Check sheet for the modelled part. Datum: model origin and axes. Units: mm. A direction names the side the tool comes from. Give positions to 0.01 mm unless a question says otherwise; leave off trailing zeros. Order: outer loops, then holes, each group sorted by start corner. A loop starts at its lowest first (then second) coordinate and runs counter-clockwise, first axis right, second up. Notation, with made-up numbers: (76, 4) -> (104, 4) arc R21 cw to (104, 13) -> close; hole circle Ø5 at (2, -5). An arc over 180 degrees is marked (long way). One line per question, with ' | ' between items. Start each with the question number.
from build123d import *

# Parameters (mm, degrees)
EXTRUDE_1_DEPTH      = 2
SKETCH_2_R           = 2.75
CUT_EXTRUDE_1_DEPTH  = 76.957158978
EXTRUDE_2_DEPTH      = 32
EXTRUDE_2_DEPTH_BACK = 2
SKETCH_3_W           = 22.737902435
SKETCH_3_H           = 2
CUT_EXTRUDE_2_DEPTH  = 83.398361634
SKETCH_7_W           = 1
SKETCH_7_H           = 2
CUT_EXTRUDE_3_DEPTH  = 2
FILLET_1_R           = 3
FILLET_2_R           = 1


with BuildPart() as part:
    # 草图1 → 凸台-拉伸1 (new body)
    with BuildSketch(Plane(origin=(0, 0, 0), x_dir=(1, 0, 0), z_dir=(0, 1, 0))):
        Polygon((0, 0), (39.728252902, 0), (70.5, -11.2), (70.5, -28.2), (35.853451717, -28.2), (0, -7.5), align=None)
    extrude(amount=EXTRUDE_1_DEPTH)

    # 草图2 → 切除-拉伸1 (cut, through all)
    with BuildSketch(Plane(origin=(0, 2, 0), x_dir=(1, 0, 0), z_dir=(0, 1, 0))):
        with Locations(Location((59, -16.7, 0), (0, 0, 270))):
            Circle(SKETCH_2_R)
    extrude(amount=-CUT_EXTRUDE_1_DEPTH, mode=Mode.SUBTRACT)

    # 草图3 → 凸台-拉伸2 (add, two sides: drawn at the far end of the back side and taken through both)
    with BuildSketch(Plane.XZ.offset(-EXTRUDE_2_DEPTH_BACK)):
        with Locations((11.368951218, -1)):
            Rectangle(SKETCH_3_W, SKETCH_3_H)
    extrude(amount=EXTRUDE_2_DEPTH + EXTRUDE_2_DEPTH_BACK)

    # 草图4 → 切除-拉伸2 (cut, through all)
    with BuildSketch(Plane(origin=(0, 0, 0), x_dir=(-1, 0, 0), z_dir=(0, 0, -1))):
        with BuildLine():
            Line((-14.987902435, -26.75), (-14.987902435, -21.25))
            ThreePointArc((-14.987902435, -21.25), (-12.737902435, -19), (-10.487902435, -21.25))
            Line((-10.487902435, -21.25), (-10.487902435, -26.75))
            ThreePointArc((-10.487902435, -26.75), (-12.737902435, -29), (-14.987902435, -26.75))
        make_face()
        with BuildLine():
            Line((-14.987902435, -12.25), (-14.987902435, -6.75))
            ThreePointArc((-14.987902435, -6.75), (-12.737902435, -4.5), (-10.487902435, -6.75))
            Line((-10.487902435, -6.75), (-10.487902435, -12.25))
            ThreePointArc((-10.487902435, -12.25), (-12.737902435, -14.5), (-14.987902435, -12.25))
        make_face()
    extrude(amount=CUT_EXTRUDE_2_DEPTH, mode=Mode.SUBTRACT)

    # 草图7 → 切除-拉伸3 (cut)
    with BuildSketch(Plane(origin=(0, 2, 0), x_dir=(1, 0, 0), z_dir=(0, 1, 0))):
        with Locations((23.237902435, -1)):
            Rectangle(SKETCH_7_W, SKETCH_7_H)
    extrude(amount=-CUT_EXTRUDE_3_DEPTH, mode=Mode.SUBTRACT)

    # 圆角1
    fillet_1_edges = [part.edges().sort_by_distance(p)[0] for p in [
        (11.368951218, 2, -2),
    ]]
    fillet(fillet_1_edges, radius=FILLET_1_R)

    # 圆角2
    fillet_2_edges = [part.edges().sort_by_distance(p)[0] for p in [
        (11.368951218, 0, 0),
    ]]
    fillet(fillet_2_edges, radius=FILLET_2_R)


solid = part.part
1. Cross-section at A-A on y = -10. Record the boundary of the cut face in (x, z), and give its area (3 significant figures).
2. Go/stop test with flat-tipped pins: pin 1 (2 mm diameter, centred on y = -9, z = -1, fed in from +X); pin 2 (6 mm diameter, centred on x = 10, y = -25.5, fed in from +Z); pin 3 (1.6 mm diameter, centred on x = 33.5, y = 1, fed in from -Z). Record where each tip stops, or that it passes through.
3. Cross-section at C-C on x = 21. Record the boundary of the cut face in (y, z).
4. Scan lines: probe 1 along Y at (x, z) = (30.5, 25); probe 2 along Z at (x, y) = (8, -11); probe 3 along X at (y, z) = (0.55, 16.7). Record each from-to range of solid material in increasing order.
5. Tool access check on faces 4 (the face through (11, -16, 0)), 5 (the face through (23.738, 1, 1)), 6 (the face through (32, 1, 0)), 7 (the face through (14.988, -24, -1)). Record the directions out of +Z, -Z, +X, -X, +Y, -Y that give a thin tool (end or side, any length) a straight path to the whole face; none if there is none.
6. Cross-section at D-D on z = 8.5. Record the boundary of the cut face in (x, y), and give its area (3 significant figures).
7. Mould release check, pull along X, two halves, no side actions. Record for faces 1 (the face through (18.178, 0.986, 17.995)), 2 (the face through (36, 0, 14)), 3 (the face through (12.7, -14.5, -1)): +X half, -X half, draft (parallel to the pull), parting line (faces both ways), or undercut.
8. Cross-section at B-B on z = 15.5. Record the boundary of the cut face in (x, y), and give its area (3 significant figures).
Response values:
1) outline: (0, -2) -> (10.49, -2) -> (10.49, 0) -> (0, 0) -> close; (14.99, -2) -> (22.74, -2) -> (22.74, 0) -> (14.99, 0) -> close | area: 36.5 mm²
2) pin 1: stops at x = 22.74 | pin 2: stops at z = 0 | pin 3: stops at z = 0
3) outline: (-32, -2) -> (-1, -2) arc R3 ccw to (2, 1) -> (2, 19.62) -> (0, 19.62) -> (0, 1) arc R1 cw to (-1, 0) -> (-32, 0) -> close
4) probe 1: y = 0 to 2 | probe 2: z = -2 to 0 | probe 3: x = 15.93 to 56.25, 61.75 to 70.5
5) face 4: +Z, +X, -X, -Y | face 5: -Z, +Y, -Y | face 6: -Z, +X, +Y, -Y | face 7: +Z, -Z
6) outline: (1.73, 0) -> (63.08, 0) -> (63.08, 2) -> (1.73, 2) -> close | area: 123 mm²
7) face 1: -X half | face 2: draft | face 3: undercut
8) outline: (13.86, 0) -> (56.53, 0) -> (56.53, 2) -> (13.86, 2) -> close; (61.47, 0) -> (70.5, 0) -> (70.5, 2) -> (61.47, 2) -> close | area: 103 mm²
